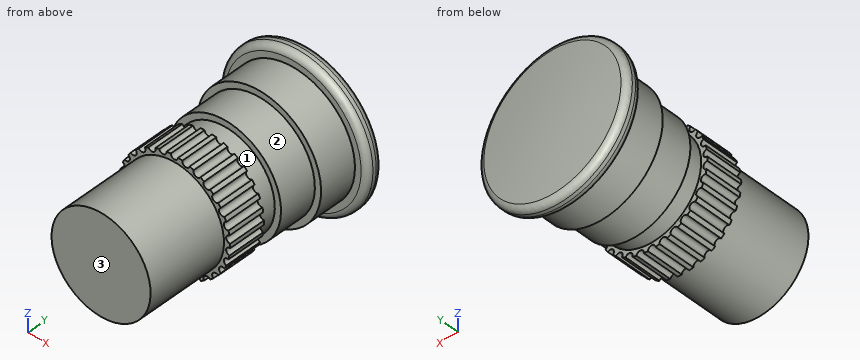
from build123d import *

# Parameters (mm, degrees)
SKETCH_3_R          = 10
EXTRUDE_1_DEPTH     = 6
SKETCH_5_R          = 9
EXTRUDE_2_DEPTH     = 6
SKETCH_7_R          = 8
EXTRUDE_3_DEPTH     = 3
SKETCH_10_R         = 9
EXTRUDE_4_DEPTH     = 6
SKETCH_11_R         = 8
EXTRUDE_5_DEPTH     = 13
FILLET_1_R          = 1
SKETCH_12_R         = 0.6
CUT_EXTRUDE_1_DEPTH = 6


with BuildPart() as part:
    # 草图1 → 旋转1 (revolve)
    with BuildSketch(Plane.XY, mode=Mode.PRIVATE) as revolve_1_sk:
        with BuildLine():
            Line((12, 0), (12, 2.5))
            ThreePointArc((12, 2.5), (6.005206075, 2.874945794), (0, 3))
            Line((0, 3), (0, 0))
            Line((0, 0), (12, 0))
        make_face()
    revolve(revolve_1_sk.sketch.rotate(Axis((0, 3, 0), (0, -1, 0)), 180), axis=Axis((0, 3, 0), (0, -1, 0)))

    # 草图3 → 凸台-拉伸1 (add)
    with BuildSketch(Plane.XZ):
        with Locations(Location((0, 0, 0), (0, 0, 270))):
            Circle(SKETCH_3_R)
    extrude(amount=EXTRUDE_1_DEPTH)

    # 草图5 → 凸台-拉伸2 (add)
    with BuildSketch(Plane.XZ.offset(6)):
        with Locations(Location((0, 0, 0), (0, 0, 270))):
            Circle(SKETCH_5_R)
    extrude(amount=EXTRUDE_2_DEPTH)

    # 草图7 → 凸台-拉伸3 (add)
    with BuildSketch(Plane.XZ.offset(12)):
        with Locations(Location((0, 0, 0), (0, 0, 270))):
            Circle(SKETCH_7_R)
    extrude(amount=EXTRUDE_3_DEPTH)

    # 草图10 → 凸台-拉伸4 (add)
    with BuildSketch(Plane.XZ.offset(15)):
        with Locations(Location((0, 0, 0), (0, 0, 270))):
            Circle(SKETCH_10_R)
    extrude(amount=EXTRUDE_4_DEPTH)

    # 草图11 → 凸台-拉伸5 (add)
    with BuildSketch(Plane.XZ.offset(21)):
        with Locations(Location((0, 0, 0), (0, 0, 270))):
            Circle(SKETCH_11_R)
    extrude(amount=EXTRUDE_5_DEPTH)

    # 圆角1
    fillet_1_edges = [part.edges().sort_by_distance(p)[0] for p in [
        (12, 0, 0),
        (12, 2.5, 0),
    ]]
    fillet(fillet_1_edges, radius=FILLET_1_R)

    # 草图12 → 切除-拉伸1 (cut)
    with BuildSketch(Plane.XZ.offset(21)):
        with Locations((0, 9)):
            Circle(SKETCH_12_R)
        with Locations((1.871205217, 8.803328407)):
            Circle(SKETCH_12_R)
        with Locations((3.660629788, 8.221909119)):
            Circle(SKETCH_12_R)
        with Locations((5.290067271, 7.281152949)):
            Circle(SKETCH_12_R)
        with Locations((6.688303429, 6.022175457)):
            Circle(SKETCH_12_R)
        with Locations((7.794228634, 4.5)):
            Circle(SKETCH_12_R)
        with Locations((8.559508647, 2.781152949)):
            Circle(SKETCH_12_R)
        with Locations((8.950697058, 0.940756169)):
            Circle(SKETCH_12_R)
        with Locations((8.950697058, -0.940756169)):
            Circle(SKETCH_12_R)
        with Locations((8.559508647, -2.781152949)):
            Circle(SKETCH_12_R)
        with Locations((7.794228634, -4.5)):
            Circle(SKETCH_12_R)
        with Locations((6.688303429, -6.022175457)):
            Circle(SKETCH_12_R)
        with Locations((5.290067271, -7.281152949)):
            Circle(SKETCH_12_R)
        with Locations((3.660629788, -8.221909119)):
            Circle(SKETCH_12_R)
        with Locations((1.871205217, -8.803328407)):
            Circle(SKETCH_12_R)
        with Locations((0, -9)):
            Circle(SKETCH_12_R)
        with Locations((-1.871205217, -8.803328407)):
            Circle(SKETCH_12_R)
        with Locations((-3.660629788, -8.221909119)):
            Circle(SKETCH_12_R)
        with Locations((-5.290067271, -7.281152949)):
            Circle(SKETCH_12_R)
        with Locations((-6.688303429, -6.022175457)):
            Circle(SKETCH_12_R)
        with Locations((-7.794228634, -4.5)):
            Circle(SKETCH_12_R)
        with Locations((-8.559508647, -2.781152949)):
            Circle(SKETCH_12_R)
        with Locations((-8.950697058, -0.940756169)):
            Circle(SKETCH_12_R)
        with Locations((-8.950697058, 0.940756169)):
            Circle(SKETCH_12_R)
        with Locations((-8.559508647, 2.781152949)):
            Circle(SKETCH_12_R)
        with Locations((-7.794228634, 4.5)):
            Circle(SKETCH_12_R)
        with Locations((-6.688303429, 6.022175457)):
            Circle(SKETCH_12_R)
        with Locations((-5.290067271, 7.281152949)):
            Circle(SKETCH_12_R)
        with Locations((-3.660629788, 8.221909119)):
            Circle(SKETCH_12_R)
        with Locations((-1.871205217, 8.803328407)):
            Circle(SKETCH_12_R)
    extrude(amount=-CUT_EXTRUDE_1_DEPTH, mode=Mode.SUBTRACT)


solid = part.part
Model file for the job. Use its own axes, mm. Face numbers are marked on the shaded views. Give positions to 0.01 mm unless a question says otherwise; leave off trailing zeros. Write each loop counter-clockwise with the first axis right and the second up, starting at its lowest first coordinate (ties: lowest second). Pieces come first, ordered by that corner, then holes. Notation, with made-up numbers: (-2.5, 30.25) - (42.5, 30.25) arc R34 ccw to (42.5, 62.25) - close; hole circle Ø4 at (-36, 66.5). An arc over 180 degrees is marked (long way). Answer as CSV lines item,"result".
1. Band-saw the part on B-B (y = -4). Write the cut outline in (x, z).
Responses:
outline,"circle Ø20 at (0, 0)"
2. Drill centre lines: L1, parallel to Z at x = -5, y = -0.5; L2, parallel to Z at x = -7.75, y = -19; L3, parallel to Y at x = 8.5, z = -8. Where is each one in solid material? Low to high. Write a range as [from, to].
Responses:
L1,"z = [-8.66, 8.66]"
L2,"z = [-3.9, 3.9]"
L3,"y = [0.26, 2.32]"
3. Band-saw the part on A-A (y = -10.5). Write the cut outline in (x, z).
Responses:
outline,"circle Ø18 at (0, 0)"
4. Two-plate mould, pull along Y, no slides. Class the marked faces 1, 2 and 3: +Y half, -Y half, draft (parallel to the pull), parting line (faces both ways), or undercut.
Responses:
face 1,"undercut"
face 2,"draft"
face 3,"-Y half"
5. Pin check, flat tips, straight feed: pin 1 (8 mm diameter, centred on x = 2.5, y = -24.5, fed in from +Z); pin 2 (1 mm diameter, centred on y = -7, z = -8.5, fed in from +X); pin 3 (1 mm diameter, centred on x = 5, y = -4.5, fed in from -Z). Stop position of each tip, or through.
Responses:
pin 1,"stops at z = 8.98"
pin 2,"stops at x = 4.12"
pin 3,"stops at z = -8.93"
